Here's how the part is built. I have some questions about the finished solid (model axes, mm). Face numbers are marked on the shaded views. Round coordinates to 2 decimals unless told otherwise and drop trailing zeros. Order: outer loops, then holes, each group sorted by start corner. A loop starts at its lowest first (then second) coordinate and runs counter-clockwise, first axis right, second up. Notation, with made-up numbers: (15.5, -34) -> (37.5, -34) arc R9 ccw to (37.5, -29) -> close; hole circle Ø4 at (-32, 69). An arc over 180 degrees is marked (long way). Use a Markdown table: item, result. Add a question column.
(1) I want a section at C-C, the plane y = -12.5. Please give me the cut outline in (x, z).
(2) If I drill on probe 1 along X at (y, z) = (-10.5, 20.5); probe 2 along X at (y, z) = (-8.5, 4); probe 3 along Z at (x, y) = (35, -21.5), over which ranges is the centre line in solid material (lowest first)?
(3) I'm going to push flat-ended pins straight in: P1, Ø6, axis at y = -15.5, z = 6.5, coming from the -X side; P2, Ø5, axis at y = -1.5, z = 18, coming from the -X side (3 decimals); P3, Ø4.5, axis at x = 17.5, z = 28.5, coming from the +Y side. Where does each tip first touch, or does it pass through?
(4) I want a section at D-D, the plane z = 12. Give the number of separate pieces and of enclosed holes in the cut face, then the cut area to 3 significant figures.
(5) Thinking about a two-plate mould opening in Y: for the marked faces 1, 2 and 3, which applies, pulls with the +Y half, pulls with the -Y half, needs draft (parallel to the pull), parting line crosses it, or undercut?
from build123d import *

# Parameters (mm, degrees)
F0_R     = 14.2875
F1_DEPTH = 25.4
F2_DEPTH = 44.45


with BuildPart() as f1:
    # F0 (on Top) → F1 (new body)
    with BuildSketch(Plane.XY):
        with BuildLine():
            ThreePointArc((-13.470384, -4.7625), (-14.2875, 0), (-13.470384, 4.7625))
            Line((-13.470384, 4.7625), (-19.05, 4.7625))
            Line((-19.05, 4.7625), (-19.05, -4.7625))
            Line((-19.05, -4.7625), (-13.470384, -4.7625))
        make_face()
        with BuildLine():
            ThreePointArc((5.042647, 28.126541), (21.916025, 18.336262), (28.575, 0))
            ThreePointArc((28.575, 0), (21.916025, -18.336262), (5.042647, -28.126541))
            Line((5.042647, -28.126541), (57.336765, -18.751028))
            ThreePointArc((57.336765, -18.751028), (34.925, 0), (57.336765, 18.751028))
            Line((57.336765, 18.751028), (5.042647, 28.126541))
        make_face()
        with BuildLine():
            ThreePointArc((5.042647, -28.126541), (21.916025, -18.336262), (28.575, 0))
            ThreePointArc((28.575, 0), (21.916025, 18.336262), (5.042647, 28.126541))
            ThreePointArc((5.042647, 28.126541), (-28.575, 0), (5.042647, -28.126541))
        make_face()
        with BuildLine():
            ThreePointArc((-13.470384, 4.7625), (0, 14.2875), (13.470384, 4.7625))
            Line((13.470384, 4.7625), (19.05, 4.7625))
            Line((19.05, 4.7625), (19.05, -4.7625))
            Line((19.05, -4.7625), (13.470384, -4.7625))
            ThreePointArc((13.470384, -4.7625), (0, -14.2875), (-13.470384, -4.7625))
            Line((-13.470384, -4.7625), (-19.05, -4.7625))
            Line((-19.05, -4.7625), (-19.05, 4.7625))
            Line((-19.05, 4.7625), (-13.470384, 4.7625))
        make_face(mode=Mode.SUBTRACT)
        with BuildLine():
            ThreePointArc((73.025, 0), (68.585683, 12.224174), (57.336765, 18.751028))
            ThreePointArc((57.336765, 18.751028), (34.925, 0), (57.336765, -18.751028))
            ThreePointArc((57.336765, -18.751028), (68.585683, -12.224174), (73.025, 0))
        make_face()
        with Locations((53.975, 0)):
            Circle(F0_R, mode=Mode.SUBTRACT)
    extrude(amount=F1_DEPTH)

    # F0 (on Top) → F2 (join)
    with BuildSketch(Plane.XY):
        with BuildLine():
            ThreePointArc((5.042647, -28.126541), (21.916025, -18.336262), (28.575, 0))
            ThreePointArc((28.575, 0), (21.916025, 18.336262), (5.042647, 28.126541))
            ThreePointArc((5.042647, 28.126541), (-28.575, 0), (5.042647, -28.126541))
        make_face()
        with BuildLine():
            ThreePointArc((-13.470384, 4.7625), (0, 14.2875), (13.470384, 4.7625))
            Line((13.470384, 4.7625), (19.05, 4.7625))
            Line((19.05, 4.7625), (19.05, -4.7625))
            Line((19.05, -4.7625), (13.470384, -4.7625))
            ThreePointArc((13.470384, -4.7625), (0, -14.2875), (-13.470384, -4.7625))
            Line((-13.470384, -4.7625), (-19.05, -4.7625))
            Line((-19.05, -4.7625), (-19.05, 4.7625))
            Line((-19.05, 4.7625), (-13.470384, 4.7625))
        make_face(mode=Mode.SUBTRACT)
        with BuildLine():
            ThreePointArc((-13.470384, -4.7625), (-14.2875, 0), (-13.470384, 4.7625))
            Line((-13.470384, 4.7625), (-19.05, 4.7625))
            Line((-19.05, 4.7625), (-19.05, -4.7625))
            Line((-19.05, -4.7625), (-13.470384, -4.7625))
        make_face()
    extrude(amount=F2_DEPTH)


solid = f1.part
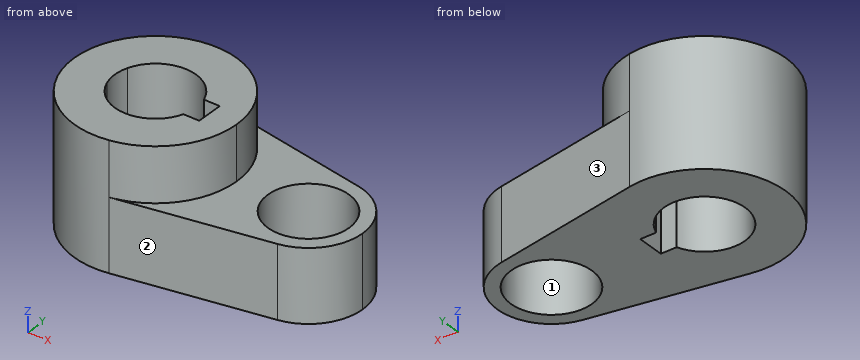
Taken from the geometry:
| question | item | result |
|---|---|---|
| 1 | outline | (-25.7, 0) -> (-6.92, 0) -> (-6.92, 44.45) -> (-25.7, 44.45) -> close; (6.92, 0) -> (47.06, 0) -> (47.06, 25.4) -> (25.7, 25.4) -> (25.7, 44.45) -> (6.92, 44.45) -> close; (60.89, 0) -> (68.35, 0) -> (68.35, 25.4) -> (60.89, 25.4) -> close |
| 2 | probe 1 | x = -26.58 to -9.69, 9.69 to 44.29, 63.66 to 69.87 |
| 2 | probe 2 | x = -27.28 to -11.48, 11.48 to 42.49, 65.46 to 71.02 |
| 2 | probe 3 | z = 0 to 25.4 |
| 3 | P1 | stops at x = -25.7 |
| 3 | P2 | stops at x = -28.575 |
| 3 | P3 | stops at y = 24.17 |
| 4 | separate pieces | 1 |
| 4 | enclosed holes | 2 |
| 4 | area | 3,130 mm2 |
| 5 | face 1 | undercut |
| 5 | face 2 | pulls with the -Y half |
| 5 | face 3 | pulls with the +Y half |
